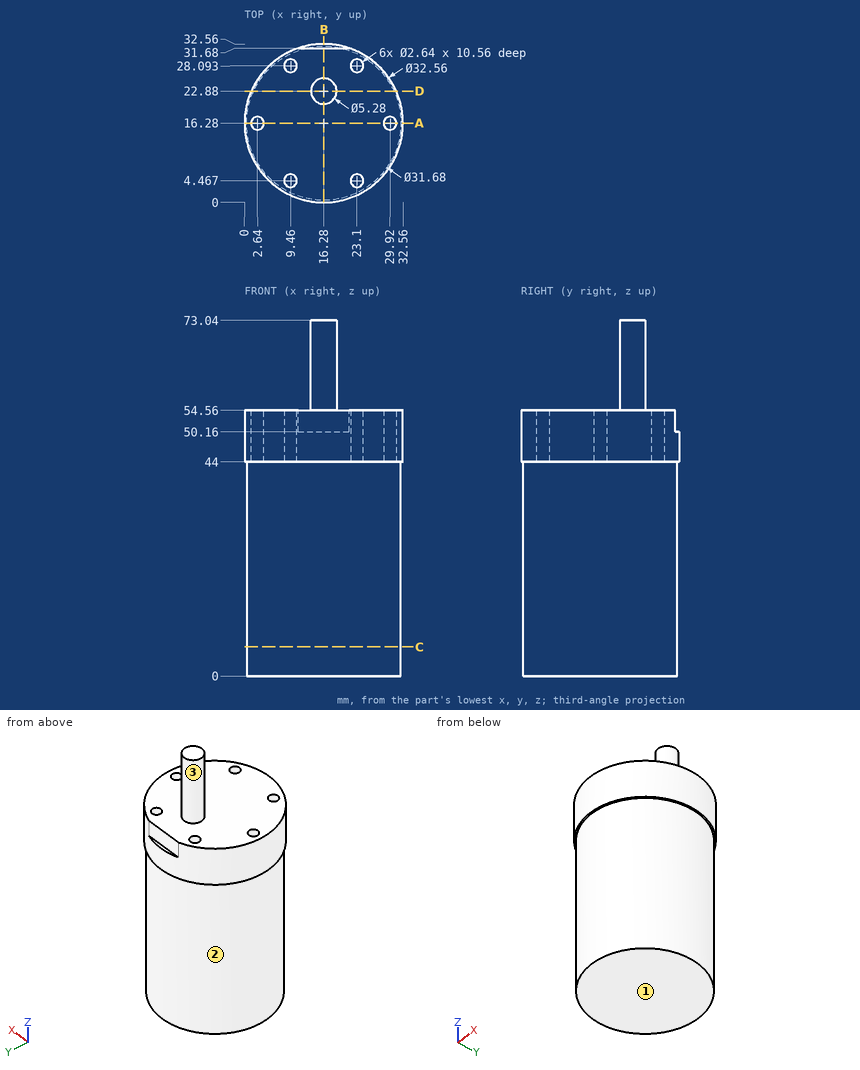
Geometry: see drawing. Coordinates: mm, zero at the bounding-box minimum. A direction names the side the tool comes from. Give positions to 0.01 mm unless a question says otherwise; leave off trailing zeros. Loops run counter-clockwise (first coordinate to the right, second up) from the corner with the lowest first, then second, coordinate; pieces in that order, holes last. Notation, with made-up numbers: (50, 78.25) -> (108, 78.25) arc R26 cw to (108, 114.25) -> close; hole circle Ø10 at (51.5, -6). An arc over 180 degrees is marked (long way). Answer as a JSON object with one key per item and string values. Group by question number.
Item 1: Pin query (flat end, axial travel): P1, Ø3, axis at x = 3, y = 16, coming from the +Z side; P2, Ø2.5, axis at x = 23.1, y = 28.09, coming from the +Z side; P3, Ø6, axis at x = 22.5, z = 56, coming from the -Y side. Return the tip coordinate at first contact, or that it passes through.
Item 2: Cut plane D-D, the plane y = 22.88. Return the cut outline in (x, z), and give its area (3 significant figures).
Item 3: Cut plane A-A, the plane y = 16.28. Return the cut outline in (x, z).
Item 4: Cut plane C-C, the plane z = 6. Return the cut outline in (x, y).
Item 5: Reachability of the marked faces 1, 2 and 3 from +Z, -Z, +X, -X, +Y, -Y: full face, straight path, thin tool, end or side. Return the list, or none.
Item 6: Cut plane B-B, the plane x = 16.28. Return the cut outline in (y, z), and give its area (3 significant figures).
Item 7: Line query: probe 1 along X at (y, z) = (16, 46); probe 2 along Z at (x, y) = (2, 17.5); probe 3 along Y at (x, z) = (9, 48) (1 decimal). Output: solid intervals per line, ascending.
Checks:
{
 "1": {"P1": "stops at z = 54.56", "P2": "stops at z = 44", "P3": "stops at y = 0.4"},
 "2": {"outline": "(1.4, 44) -> (1.88, 44) -> (1.88, 0) -> (30.68, 0) -> (30.68, 44) -> (31.16, 44) -> (31.16, 54.56) -> (18.92, 54.56) -> (18.92, 73.04) -> (13.64, 73.04) -> (13.64, 54.56) -> (1.4, 54.56) -> close", "area": "1,680 mm²"},
 "3": {"outline": "(0, 44) -> (0.44, 44) -> (0.44, 0) -> (32.12, 0) -> (32.12, 44) -> (32.56, 44) -> (32.56, 54.56) -> (31.24, 54.56) -> (31.24, 44) -> (28.6, 44) -> (28.6, 54.56) -> (3.96, 54.56) -> (3.96, 44) -> (1.32, 44) -> (1.32, 54.56) -> (0, 54.56) -> close"},
 "4": {"outline": "circle Ø31.68 at (16.28, 16.28)"},
 "5": {"face 1": "-Z, +X, -X, +Y, -Y", "face 2": "-Z", "face 3": "+Z"},
 "6": {"outline": "(0, 44) -> (0.44, 44) -> (0.44, 0) -> (32.12, 0) -> (32.12, 44) -> (32.56, 44) -> (32.56, 50.16) -> (31.68, 50.16) -> (31.68, 54.56) -> (25.52, 54.56) -> (25.52, 73.04) -> (20.24, 73.04) -> (20.24, 54.56) -> (0, 54.56) -> close", "area": "1,830 mm²"},
 "7": {"probe 1": "x = 0 to 1.35, 3.93 to 28.63, 31.21 to 32.56", "probe 2": "z = 0 to 54.56", "probe 3": "y = 1.7 to 3.2, 5.7 to 26.9, 29.3 to 30.8"}
}
